Geometry check sheet. Reference: drawing and pictorial views, mm from the part's lowest x, y, z. A direction names the side the tool comes from. Round coordinates to 2 decimals unless told otherwise and drop trailing zeros. Write each loop counter-clockwise with the first axis right and the second up, starting at its lowest first coordinate (ties: lowest second). Pieces come first, ordered by that corner, then holes. Notation, with made-up numbers: M 1,76 L 6,76 A25 ccw 6,106 Z; hole C 7.25,84 d3. An arc over 180 degrees is marked long. One line per question, with ' | ' between items.
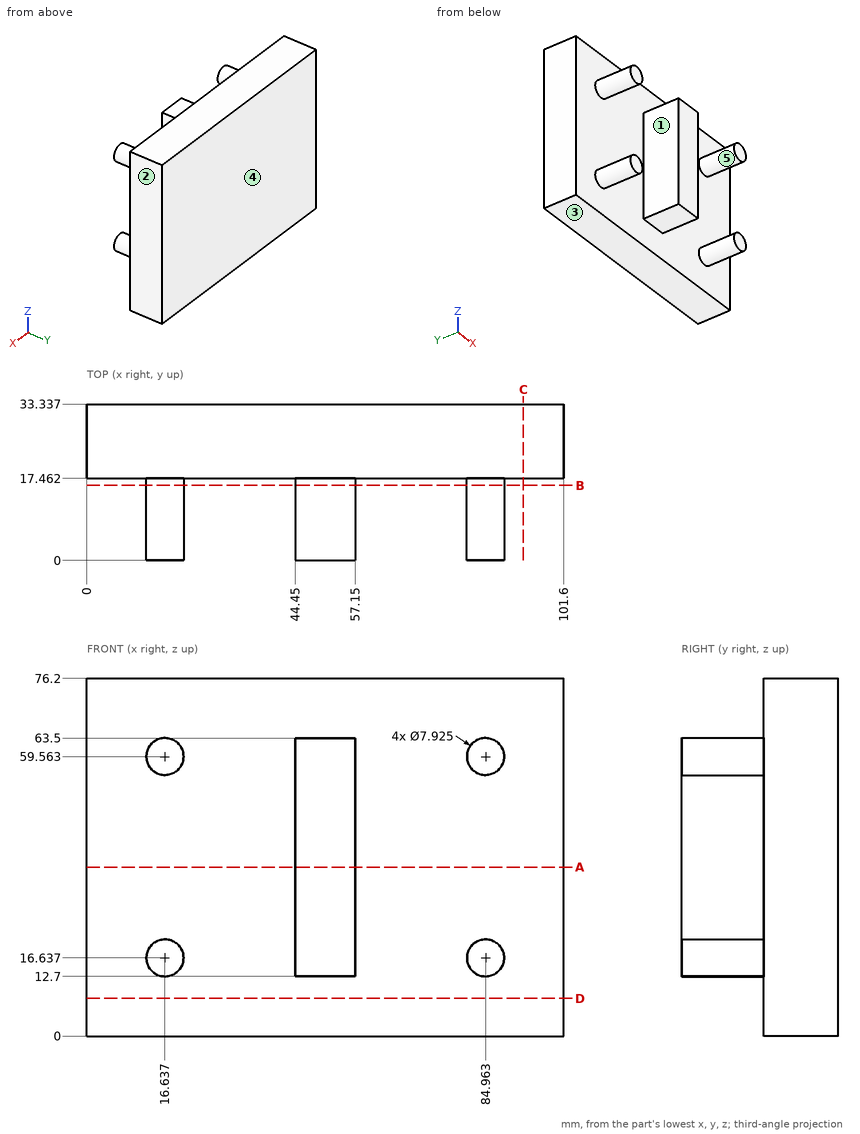
1. Tool access check on the marked faces 4 and 5. Record the directions out of +Z, -Z, +X, -X, +Y, -Y that give a thin tool (end or side, any length) a straight path to the whole face; none if there is none.
Results:
face 4: +Z, -Z, +X, -X, +Y | face 5: -Y
2. Section check B-B, the plane y = 16. Count the separate pieces of the cut face and the enclosed holes in it.
Results:
separate pieces: 5 | enclosed holes: 0
3. Section check D-D, the plane z = 8. Record the cut outline in (x, y), then the cut area to 3 significant figures.
Results:
outline: M 0,17.46 L 101.6,17.46 L 101.6,33.34 L 0,33.34 Z | area: 1,610 mm2
4. Section check C-C, the plane x = 93. Record the cut outline in (y, z).
Results:
outline: M 17.46,0 L 33.34,0 L 33.34,76.2 L 17.46,76.2 Z
5. Section check A-A, the plane z = 36. Record the cut outline in (x, y).
Results:
outline: M 0,17.46 L 44.45,17.46 L 44.45,0 L 57.15,0 L 57.15,17.46 L 101.6,17.46 L 101.6,33.34 L 0,33.34 Z
6. Mould release check, pull along X, two halves, no side actions. Record for the marked faces 1, 2 and 3: pulls with the +X half, pulls with the -X half, needs draft (parallel to the pull), parting line crosses it, or undercut.
Results:
face 1: undercut | face 2: pulls with the +X half | face 3: needs draft
7. Go/stop test with flat-tipped pins: P1, Ø4, axis at x = 18, y = 7, coming from the +Z side (1 decimal); P2, Ø3, axis at y = 24.5, z = 37.5, coming from the -X side; P3, Ø19, axis at y = 7.5, z = 31, coming from the +X side; P4, Ø19, axis at y = 5, z = 43, coming from the -X side. Record where each tip stops, or that it passes through.
Results:
P1: stops at z = 63.5 | P2: stops at x = 0 | P3: stops at x = 57.15 | P4: stops at x = 44.45
8. Thickness scan on line 1 (X direction, y = 12, z = 39); line 2 (Y direction, x = 74.5, z = 64); line 3 (Z direction, x = 83.5, y = 16) (1 decimal). Record the ranges inside material, lowest first.
Results:
line 1: x = 44.45 to 57.15 | line 2: y = 17.46 to 33.34 | line 3: z = 13 to 20.3, 55.9 to 63.2
